from build123d import *

# Parameters (mm, degrees)
F0_R     = 3.175
F1_DEPTH = 3.048
F2_DEPTH = 6.35


with BuildPart() as f1:
    # F0 (on Front) → F1 (new body)
    with BuildSketch(Plane.XZ):
        with BuildLine():
            Line((-9.450293, 115.490625), (-15.750488, 65.484375))
            ThreePointArc((-15.750488, 65.484375), (0, 79.375), (15.750488, 65.484375))
            Line((15.750488, 65.484375), (9.450293, 115.490625))
            ThreePointArc((9.450293, 115.490625), (9.506305, 114.896483), (9.525, 114.3))
            ThreePointArc((9.525, 114.3), (-0.596483, 104.793695), (-9.450293, 115.490625))
        make_face()
        with Locations((-3.175, 100.0252)):
            Circle(F0_R, mode=Mode.SUBTRACT)
        with BuildLine():
            ThreePointArc((-9.477255, -0.9525), (-0.476848, 9.513056), (9.525, 0))
            ThreePointArc((9.525, 0), (6.854408, -6.613827), (0.340179, -9.518923))
            Line((0.340179, -9.518923), (44.733482, -7.932436))
            ThreePointArc((44.733482, -7.932436), (36.512502, -0.006243), (44.721004, 7.932872))
            Line((44.721004, 7.932872), (18.967926, 8.812653))
            ThreePointArc((18.967926, 8.812653), (13.25428, 11.525202), (11.328669, 17.549793))
            Line((11.328669, 17.549793), (15.675725, 60.99256))
            ThreePointArc((15.675725, 60.99256), (-0.463847, 47.631778), (-15.795426, 61.9125))
            Line((-15.795426, 61.9125), (-9.477255, -0.9525))
        make_face()
        with BuildLine():
            ThreePointArc((9.450293, 115.490625), (0, 123.825), (-9.450293, 115.490625))
            ThreePointArc((-9.450293, 115.490625), (-0.596483, 104.793695), (9.525, 114.3))
            ThreePointArc((9.525, 114.3), (9.506305, 114.896483), (9.450293, 115.490625))
        make_face()
        with Locations((0, 114.3)):
            Circle(F0_R, mode=Mode.SUBTRACT)
        with BuildLine():
            ThreePointArc((-15.750488, 65.484375), (-15.873744, 63.699705), (-15.795426, 61.9125))
            ThreePointArc((-15.795426, 61.9125), (-0.463847, 47.631778), (15.675725, 60.99256))
            Line((15.675725, 60.99256), (15.861756, 62.851674))
            ThreePointArc((15.861756, 62.851674), (15.871689, 63.175769), (15.875, 63.5))
            ThreePointArc((15.875, 63.5), (15.843841, 64.494139), (15.750488, 65.484375))
            ThreePointArc((15.750488, 65.484375), (0, 79.375), (-15.750488, 65.484375))
        make_face()
        with Locations((0, 63.5)):
            Circle(F0_R, mode=Mode.SUBTRACT)
        with BuildLine():
            ThreePointArc((0.340179, -9.518923), (6.854408, -6.613827), (9.525, 0))
            ThreePointArc((9.525, 0), (-0.476848, 9.513056), (-9.477255, -0.9525))
            ThreePointArc((-9.477255, -0.9525), (-6.262383, -7.17692), (0.340179, -9.518923))
        make_face()
        Circle(F0_R, mode=Mode.SUBTRACT)
        with BuildLine():
            ThreePointArc((44.721004, 7.932872), (36.512502, -0.006243), (44.733482, -7.932436))
            ThreePointArc((44.733482, -7.932436), (50.162007, -5.511523), (52.3875, 0))
            ThreePointArc((52.3875, 0), (50.15767, 5.516014), (44.721004, 7.932872))
        make_face()
        with Locations((44.45, 0)):
            Circle(F0_R, mode=Mode.SUBTRACT)
    extrude(amount=F1_DEPTH)

    # F0 (on Front) → F2 (join)
    with BuildSketch(Plane.XZ):
        with BuildLine():
            ThreePointArc((44.721004, 7.932872), (36.512502, -0.006243), (44.733482, -7.932436))
            ThreePointArc((44.733482, -7.932436), (50.162007, -5.511523), (52.3875, 0))
            ThreePointArc((52.3875, 0), (50.15767, 5.516014), (44.721004, 7.932872))
        make_face()
        with Locations((44.45, 0)):
            Circle(F0_R, mode=Mode.SUBTRACT)
        with BuildLine():
            ThreePointArc((0.340179, -9.518923), (6.854408, -6.613827), (9.525, 0))
            ThreePointArc((9.525, 0), (-0.476848, 9.513056), (-9.477255, -0.9525))
            ThreePointArc((-9.477255, -0.9525), (-6.262383, -7.17692), (0.340179, -9.518923))
        make_face()
        Circle(F0_R, mode=Mode.SUBTRACT)
        with BuildLine():
            ThreePointArc((-15.750488, 65.484375), (-15.873744, 63.699705), (-15.795426, 61.9125))
            ThreePointArc((-15.795426, 61.9125), (-0.463847, 47.631778), (15.675725, 60.99256))
            Line((15.675725, 60.99256), (15.861756, 62.851674))
            ThreePointArc((15.861756, 62.851674), (15.871689, 63.175769), (15.875, 63.5))
            ThreePointArc((15.875, 63.5), (15.843841, 64.494139), (15.750488, 65.484375))
            ThreePointArc((15.750488, 65.484375), (0, 79.375), (-15.750488, 65.484375))
        make_face()
        with Locations((0, 63.5)):
            Circle(F0_R, mode=Mode.SUBTRACT)
        with BuildLine():
            ThreePointArc((9.450293, 115.490625), (0, 123.825), (-9.450293, 115.490625))
            ThreePointArc((-9.450293, 115.490625), (-0.596483, 104.793695), (9.525, 114.3))
            ThreePointArc((9.525, 114.3), (9.506305, 114.896483), (9.450293, 115.490625))
        make_face()
        with Locations((0, 114.3)):
            Circle(F0_R, mode=Mode.SUBTRACT)
    extrude(amount=-F2_DEPTH)


solid = f1.part
Design review of the part built by this model. Coordinates are the model's own, in mm. A direction names the side the tool comes from. Coordinates: 2 decimals unless noted, no trailing zeros. Loops run counter-clockwise (first coordinate to the right, second up) from the corner with the lowest first, then second, coordinate; pieces in that order, holes last.
Item 1: Add section B-B (x = 39). Write out the cut boundary in (y, z).
Completed:
outline: (-3.05, -8.14) - (0, -8.14) - (0, -5.77) - (6.35, -5.77) - (6.35, 5.77) - (0, 5.77) - (0, 8.13) - (-3.05, 8.13) - close
Item 2: For faces 5 (the cylindrical face through (-3.588, -1.503, 103.173)), 6 (the flat face through (5, 0, 21)), list the 3-axis set-ups (+Z, -Z, +X, -X, +Y, -Y) from which the entire face can be reached by the end or side of a thin tool; tool diameter is ignored.
Completed:
face 5: +Y, -Y
face 6: +Y
Item 3: Draft analysis for pull direction Z (two halves, no side actions). For faces 1 (the flat face through (-12.68, -1.5, 30.92)), 2 (the flat face through (12.644, -1.503, 90.137)), 3 (the flat face through (0, 0, 91)), 4 (the flat face through (0, 6.35, 60)), state which applies: pulls with the +Z half, pulls with the -Z half, needs draft (parallel to the pull), parting line crosses it, or undercut.
Completed:
face 1: pulls with the -Z half
face 2: pulls with the +Z half
face 3: undercut
face 4: needs draft
Item 4: Add section C-C (z = 45.5). Write out the cut boundary in (x, y).
Completed:
outline: (-14.15, -3.05) - (14.13, -3.05) - (14.13, 0) - (-14.15, 0) - close
Item 5: Add section D-D (x = 32). Write out the cut boundary in (y, z).
Completed:
outline: (-3.05, -8.39) - (0, -8.39) - (0, 8.37) - (-3.05, 8.37) - close
Item 6: Wall thickness on L1, parallel to Z at x = 0, y = 2.75 (3 decimals); L2, parallel to Z at x = 6.5, y = 3.75; L3, parallel to Y at x = 30.5, z = 2.5: over which ranges is each line inside the solid? List them lowest first.
Completed:
L1: z = -9.525 to -3.175, 3.175 to 9.525, 47.625 to 60.325, 66.675 to 79.375, 104.775 to 111.125, 117.475 to 123.825
L2: z = -6.96 to 6.96, 49.02 to 77.98, 107.34 to 121.26
L3: y = -3.05 to 0
Item 7: Add section A-A (y = 2). Give the number of separate pieces and of enclosed holes in the cut face, and give its area (3 significant figures).
Completed:
separate pieces: 4
enclosed holes: 4
area: 1,430 mm2
Item 8: Clearance check with flat-ended pins moving along their axes: pin 1 (4 mm diameter, centred on x = 42.5, y = 3, fed in from -Z); pin 2 (4 mm diameter, centred on x = 36, y = -1.5, fed in from -Z); pin 3 (3 mm diameter, centred on x = 30.5, y = -2, fed in from -Z). State where each tip first meets the part, or that it passes through.
Completed:
pin 1: stops at z = -7.94
pin 2: stops at z = -8.32
pin 3: stops at z = -8.49
